Input: part model. Units: mm. Frame: model coordinates. A direction names the side the tool comes from. Give positions to 0.01 mm unless a question says otherwise; leave off trailing zeros. Order: outer loops, then holes, each group sorted by start corner. A loop starts at its lowest first (then second) coordinate and runs counter-clockwise, first axis right, second up. Notation, with made-up numbers: (22, -13) - (56, -13) arc R23 ccw to (56, 10) - close; hole circle Ø8 at (44.5, 56.25). An arc over 180 degrees is marked (long way). Use a Markdown table: item, result.
from build123d import *

# Parameters (mm, degrees)
SKETCH_1_W          = 50
SKETCH_1_H          = 30
EXTRUDE_1_DEPTH     = 5
SKETCH_2_R          = 1.25
CUT_EXTRUDE_1_DEPTH = 30.580398915
SKETCH_3_R          = 1.5
CUT_EXTRUDE_2_DEPTH = 30.580398915
SKETCH_4_W          = 11
SKETCH_4_H          = 13.5
EXTRUDE_2_DEPTH     = 10
SKETCH_5_R          = 1.5
CUT_EXTRUDE_3_DEPTH = 33.787192622
FILLET_1_R          = 2
SKETCH_6_R          = 3
CUT_EXTRUDE_4_DEPTH = 3


with BuildPart() as part:
    # Эскиз1 → Бобышка-Вытянуть1 (new body)
    with BuildSketch(Plane(origin=(0, 0, 0), x_dir=(1, 0, 0), z_dir=(0, 1, 0))):
        Rectangle(SKETCH_1_W, SKETCH_1_H)
    extrude(amount=EXTRUDE_1_DEPTH)

    # Эскиз2 → Вырез-Вытянуть1 (cut, through all)
    with BuildSketch(Plane(origin=(0, 5, 0), x_dir=(1, 0, 0), z_dir=(0, 1, 0))):
        with Locations(Location((0, 5, 0), (0, 0, 270))):
            Circle(SKETCH_2_R)
    extrude(amount=-CUT_EXTRUDE_1_DEPTH, mode=Mode.SUBTRACT)

    # Эскиз3 → Вырез-Вытянуть2 (cut, through all)
    with BuildSketch(Plane.XZ):
        with Locations(Location((-21.25, 0, 0), (0, 0, 270))):
            Circle(SKETCH_3_R)
        with Locations(Location((0, 7.5, 0), (0, 0, 270))):
            Circle(SKETCH_3_R)
        with Locations(Location((21.25, 0, 0), (0, 0, 270))):
            Circle(SKETCH_3_R)
        with Locations(Location((0, -12.5, 0), (0, 0, 270))):
            Circle(SKETCH_3_R)
    extrude(amount=-CUT_EXTRUDE_2_DEPTH, mode=Mode.SUBTRACT)

    # Эскиз4 → Бобышка-Вытянуть2 (add)
    with BuildSketch(Plane.XZ):
        with Locations((-12.5, 8.25)):
            Rectangle(SKETCH_4_W, SKETCH_4_H)
        with Locations((12.5, 8.25)):
            Rectangle(SKETCH_4_W, SKETCH_4_H)
    extrude(amount=EXTRUDE_2_DEPTH)

    # Эскиз5 → Вырез-Вытянуть3 (cut, through all)
    with BuildSketch(Plane(origin=(0, 5, 0), x_dir=(1, 0, 0), z_dir=(0, 1, 0))):
        with Locations(Location((-21.25, -10, 0), (0, 0, 270))):
            Circle(SKETCH_5_R)
        with Locations(Location((-21.25, 10, 0), (0, 0, 270))):
            Circle(SKETCH_5_R)
        with Locations(Location((21.25, -10, 0), (0, 0, 270))):
            Circle(SKETCH_5_R)
        with Locations(Location((21.25, 10, 0), (0, 0, 270))):
            Circle(SKETCH_5_R)
    extrude(amount=-CUT_EXTRUDE_3_DEPTH, mode=Mode.SUBTRACT)

    # Скругление1
    # the kernel refuses this fillet: 2 mm, written as the material it takes off along each edge
    with BuildSketch(Plane(origin=(23, 3, -13), x_dir=(0, 1, 0), z_dir=(1, 0, 0))) as fillet_1_piece_1_section:
        Polygon((0, 0), (FILLET_1_R, 0), (FILLET_1_R, -FILLET_1_R), (0, -FILLET_1_R), align=None)
    fillet_1_piece_1 = extrude(amount=FILLET_1_R, mode=Mode.PRIVATE)
    fillet_1_piece_1 = fillet_1_piece_1 - Plane(origin=(23, 3, -13), x_dir=(0, -0.7071067811865475, 0.7071067811865475), z_dir=(1, 0, 0)) * Sphere(FILLET_1_R, mode=Mode.PRIVATE)
    add(fillet_1_piece_1, mode=Mode.SUBTRACT)
    with BuildSketch(Plane(origin=(23, 3, 13), x_dir=(1, 0, 0), z_dir=(0, 0, 1))) as fillet_1_piece_2_section:
        Polygon((0, 0), (FILLET_1_R, 0), (FILLET_1_R, FILLET_1_R), (0, FILLET_1_R), align=None)
    fillet_1_piece_2 = extrude(amount=FILLET_1_R, mode=Mode.PRIVATE)
    fillet_1_piece_2 = fillet_1_piece_2 - Plane(origin=(23, 3, 13), x_dir=(-0.7071067811865475, -0.7071067811865475, 0), z_dir=(0, 0, 1)) * Sphere(FILLET_1_R, mode=Mode.PRIVATE)
    add(fillet_1_piece_2, mode=Mode.SUBTRACT)
    with BuildSketch(Plane(origin=(-23, 3, -13), x_dir=(0, 1, 0), z_dir=(-1, 0, 0))) as fillet_1_piece_3_section:
        Polygon((0, 0), (FILLET_1_R, 0), (FILLET_1_R, FILLET_1_R), (0, FILLET_1_R), align=None)
    fillet_1_piece_3 = extrude(amount=FILLET_1_R, mode=Mode.PRIVATE)
    fillet_1_piece_3 = fillet_1_piece_3 - Plane(origin=(-23, 3, -13), x_dir=(0, -0.7071067811865475, 0.7071067811865475), z_dir=(-1, 0, 0)) * Sphere(FILLET_1_R, mode=Mode.PRIVATE)
    add(fillet_1_piece_3, mode=Mode.SUBTRACT)
    with BuildSketch(Plane(origin=(-23, 3, 13), x_dir=(0, 1, 0), z_dir=(0, 0, 1))) as fillet_1_piece_4_section:
        Polygon((0, 0), (FILLET_1_R, 0), (FILLET_1_R, FILLET_1_R), (0, FILLET_1_R), align=None)
    fillet_1_piece_4 = extrude(amount=FILLET_1_R, mode=Mode.PRIVATE)
    fillet_1_piece_4 = fillet_1_piece_4 - Plane(origin=(-23, 3, 13), x_dir=(0.7071067811865475, -0.7071067811865475, 0), z_dir=(0, 0, 1)) * Sphere(FILLET_1_R, mode=Mode.PRIVATE)
    add(fillet_1_piece_4, mode=Mode.SUBTRACT)
    with BuildSketch(Plane(origin=(25, 5, -13), x_dir=(0, -1, 0), z_dir=(0, 0, 1))) as fillet_1_piece_5:
        with BuildLine():
            CenterArc((FILLET_1_R, -FILLET_1_R), FILLET_1_R, 90, 90)
            Line((0, -FILLET_1_R), (0, 0))
            Line((0, 0), (FILLET_1_R, 0))
        make_face()
    extrude(amount=26, mode=Mode.SUBTRACT)
    with BuildSketch(Plane(origin=(-23, 5, -15), x_dir=(0, 0, 1), z_dir=(1, 0, 0))) as fillet_1_piece_6:
        with BuildLine():
            CenterArc((FILLET_1_R, FILLET_1_R), FILLET_1_R, 180, 90)
            Line((0, FILLET_1_R), (0, 0))
            Line((0, 0), (FILLET_1_R, 0))
        make_face()
    extrude(amount=46, mode=Mode.SUBTRACT)
    with BuildSketch(Plane(origin=(-25, 5, 13), x_dir=(1, 0, 0), z_dir=(0, 0, -1))) as fillet_1_piece_7:
        with BuildLine():
            CenterArc((FILLET_1_R, FILLET_1_R), FILLET_1_R, 180, 90)
            Line((0, FILLET_1_R), (0, 0))
            Line((0, 0), (FILLET_1_R, 0))
        make_face()
    extrude(amount=26, mode=Mode.SUBTRACT)
    with BuildSketch(Plane(origin=(-25, -5, -15), x_dir=(0, 0, 1), z_dir=(0, 1, 0)), Plane(origin=(-25, -5, 15), x_dir=(1, 0, 0), z_dir=(0, 1, 0))) as fillet_1_piece_8:
        with BuildLine():
            CenterArc((FILLET_1_R, FILLET_1_R), FILLET_1_R, 180, 90)
            Line((0, FILLET_1_R), (0, 0))
            Line((0, 0), (FILLET_1_R, 0))
        make_face()
    extrude(amount=8, mode=Mode.SUBTRACT)
    with BuildSketch(Plane(origin=(25, -5, -15), x_dir=(0, 0, 1), z_dir=(0, 1, 0)), Plane(origin=(25, -5, 15), x_dir=(-1, 0, 0), z_dir=(0, 1, 0))) as fillet_1_piece_9:
        with BuildLine():
            CenterArc((FILLET_1_R, -FILLET_1_R), FILLET_1_R, 90, 90)
            Line((0, -FILLET_1_R), (0, 0))
            Line((0, 0), (FILLET_1_R, 0))
        make_face()
    extrude(amount=8, mode=Mode.SUBTRACT)
    with BuildSketch(Plane(origin=(23, 5, 15), x_dir=(0, -1, 0), z_dir=(-1, 0, 0))) as fillet_1_piece_10:
        with BuildLine():
            CenterArc((FILLET_1_R, -FILLET_1_R), FILLET_1_R, 90, 90)
            Line((0, -FILLET_1_R), (0, 0))
            Line((0, 0), (FILLET_1_R, 0))
        make_face()
    extrude(amount=46, mode=Mode.SUBTRACT)

    # Эскиз6 → Вырез-Вытянуть4 (cut)
    with BuildSketch(Plane(origin=(0, 5, 0), x_dir=(1, 0, 0), z_dir=(0, 1, 0))):
        with Locations(Location((0, 5, 0), (0, 0, 270))):
            Circle(SKETCH_6_R)
    extrude(amount=-CUT_EXTRUDE_4_DEPTH, mode=Mode.SUBTRACT)


solid = part.part
1. Section query D-D (x = 10.5). Return loops of the section in (y, z), then the cut area to 3 significant figures.
Response:
| item | result |
|---|---|
| outline | (-10, 1.5) - (0, 1.5) - (0, -15) - (3, -15) arc R2 ccw to (5, -13) - (5, 13) arc R2 ccw to (3, 15) - (-10, 15) - close |
| area | 283 mm^2 |
2. Section query B-B (x = -21.25). Return loops of the section in (y, z), then the cut area to 3 significant figures.
Response:
| item | result |
|---|---|
| outline | (0, -15) - (3, -15) arc R2 ccw to (5, -13) - (5, -11.5) - (0, -11.5) - close; (0, -8.5) - (5, -8.5) - (5, -1.5) - (0, -1.5) - close; (0, 1.5) - (5, 1.5) - (5, 8.5) - (0, 8.5) - close; (0, 11.5) - (5, 11.5) - (5, 13) arc R2 ccw to (3, 15) - (0, 15) - close |
| area | 103 mm^2 |
3. Section query A-A (z = -5). Return loops of the section in (x, y).
Response:
| item | result |
|---|---|
| outline | (-25, 0) - (-1.25, 0) - (-1.25, 2) - (-3, 2) - (-3, 5) - (-23, 5) arc R2 ccw to (-25, 3) - close; (1.25, 0) - (25, 0) - (25, 3) arc R2 ccw to (23, 5) - (3, 5) - (3, 2) - (1.25, 2) - close |
4. Set-up query: faces 1 (the face through (-1, 2, -4)), 2 (the face through (18, -5, 8)), 3 (the face through (-13, -10, 8)), 4 (the face through (22.515, 2.465, -0.806)), 5 (the face through (-18, -5, 8)). Return all of +Z, -Z, +X, -X, +Y, -Y with unobstructed straight access to the full face (end or side cutting, diameter ignored); none if empty.
Response:
| item | result |
|---|---|
| face 1 | +Y |
| face 2 | +Z, -Z, +X, -Y |
| face 3 | +Z, -Z, +X, -X, -Y |
| face 4 | +Y, -Y |
| face 5 | +Z, -Z, -X, -Y |
5. Mould query, pull axis Z, two halves, no side actions, for faces 6 (the face through (0.05, 1.01, -6.25)), 7 (the face through (0, 1, 15)), 8 (the face through (7, -5, 8)). Classes: pulls with the +Z half, pulls with the -Z half, needs draft (parallel to the pull), parting line crosses it, or undercut.
Response:
| item | result |
|---|---|
| face 6 | undercut |
| face 7 | pulls with the +Z half |
| face 8 | needs draft |
6. Section query C-C (y = -2). Return loops of the section in (x, z).
Response:
| item | result |
|---|---|
| outline | (-18, 1.5) - (-7, 1.5) - (-7, 15) - (-18, 15) - close; (7, 1.5) - (18, 1.5) - (18, 15) - (7, 15) - close |
7. Material intervals for line 1 along X through (y, z) = (1.65, 10); line 2 along X through (y, z) = (1.75, 7.5); line 3 along X through (y, z) = (-2.75, 2.5), sorted ascending.
Response:
| item | result |
|---|---|
| line 1 | x = -25 to -22.75, -19.75 to 19.75, 22.75 to 25 |
| line 2 | x = -25 to -1.5, 1.5 to 25 |
| line 3 | x = -18 to -7, 7 to 18 |
8. Pin query (flat end, axial travel): pin 1 (5 mm diameter, centred on x = 14.5, y = -6, fed in from -Z); pin 2 (1 mm diameter, centred on x = -16.5, z = -2.5, fed in from -Y); pin 3 (3 mm diameter, centred on y = -3, z = 9, fed in from -X). Return the tip coordinate at first contact, or that it passes through.
Response:
| item | result |
|---|---|
| pin 1 | stops at z = 1.5 |
| pin 2 | stops at y = 0 |
| pin 3 | stops at x = -18 |
